Part print with two shaded views. Sizes in mm from the minimum x, y, z corner. Round coordinates to 2 decimals unless told otherwise and drop trailing zeros. Loops run counter-clockwise (first coordinate to the right, second up) from the corner with the lowest first, then second, coordinate; pieces in that order, holes last. Notation, with made-up numbers: (15.25, -22) - (25.25, -22) arc R14 ccw to (25.25, -6) - close; hole circle Ø5 at (81, -28.75). An arc over 180 degrees is marked (long way). One line per question, with ' | ' between items.
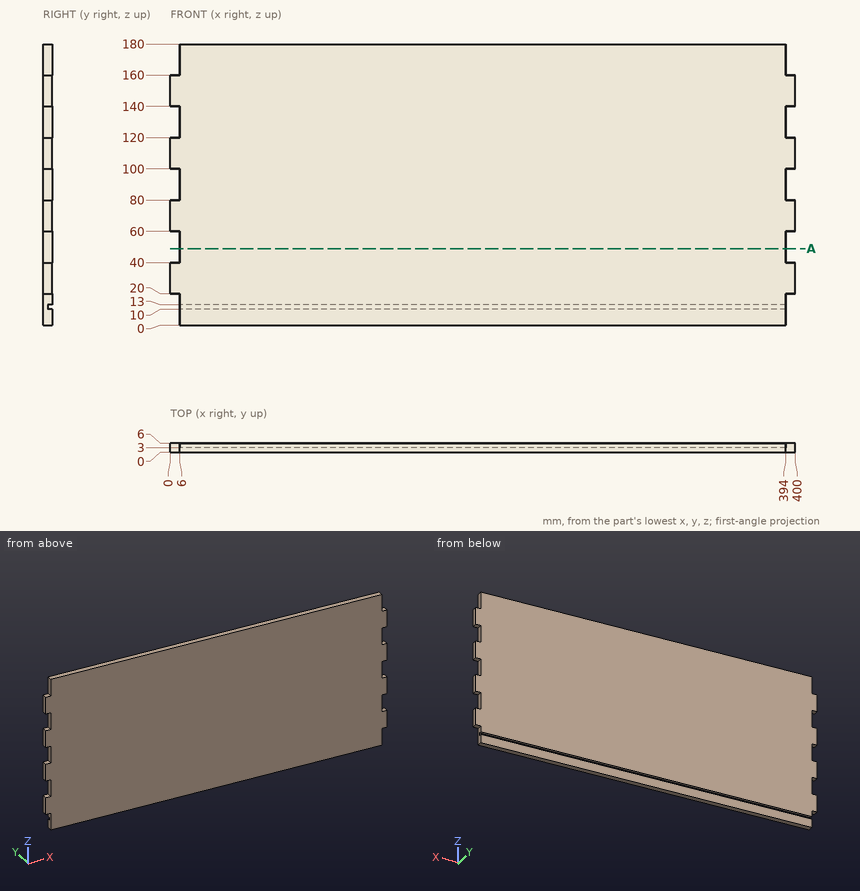
(1) Drop flat-ended pins along their axis: P1, Ø1.8, axis at x = 398.5, y = 4.5, coming from the +Z side; P2, Ø1.8, axis at x = 398, y = 4, coming from the -Z side; P3, Ø3, axis at y = 3.5, z = 128, coming from the -X side. Give the stop position or say it passes through.
Results found:
P1: stops at z = 160 | P2: stops at z = 20 | P3: stops at x = 6
(2) Probe L1, parallel to Z at x = 375.5, y = 3.5; L2, parallel to X at y = 1.7, z = 131; L3, parallel to Y at x = 116, z = 12. List the from-to ranges inside material, lowest first.
Results found:
L1: z = 0 to 10, 13 to 180 | L2: x = 6 to 394 | L3: y = 0 to 3
(3) Cut at A-A, the plane z = 49. Write the cut outline in (x, y).
Results found:
outline: (6, 0) - (394, 0) - (394, 6) - (6, 6) - close
